For this review, take the finished solid that the model builds, in its own axes (mm). Face numbers are marked on the shaded views. A direction names the side the tool comes from. Round coordinates to 2 decimals unless told otherwise and drop trailing zeros. Order: outer loops, then holes, each group sorted by start corner. A loop starts at its lowest first (then second) coordinate and runs counter-clockwise, first axis right, second up. Notation, with made-up numbers: M 76.5,13 L 117.5,13 A24 cw 117.5,25 Z; hole C -11.75,79 d10. An arc over 180 degrees is marked long. Use a Markdown table: item, result.
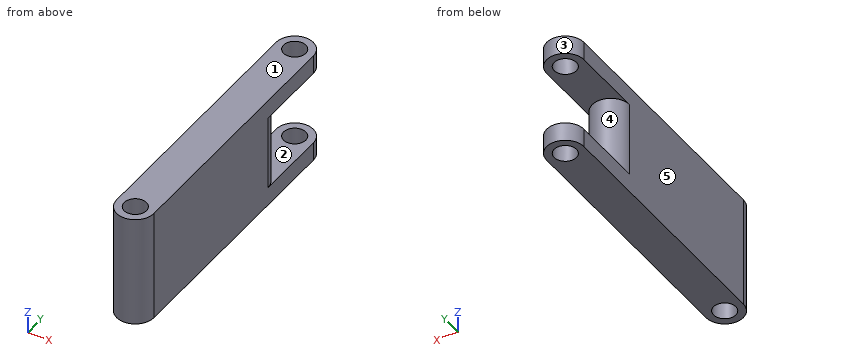
from build123d import *

# Parameters (mm, degrees)
SKETCH1_W           = 12.7
SKETCH1_H           = 101.6
BOSS_EXTRUDE1_DEPTH = 19.05
FILLET2_RADIUS      = 6.35
FILLET2_LENGTH      = 38.1
SKETCH2_R           = 3.81
CUT_EXTRUDE1_DEPTH  = 38.1
FILLET3_RADIUS      = 6.35
FILLET3_LENGTH      = 38.1
SKETCH3_W           = 25.4
SKETCH3_H           = 25.4
CUT_EXTRUDE2_DEPTH  = 56.72102386
FILLET4_RADIUS      = 6.35
FILLET4_LENGTH      = 25.4


with BuildPart() as part:
    # Sketch1 → Boss-Extrude1 (new, symmetric)
    with BuildSketch(Plane.XY):
        Rectangle(SKETCH1_W, SKETCH1_H)
    extrude(amount=BOSS_EXTRUDE1_DEPTH, both=True)

    # Fillet2: full round fillet: the end face becomes a half cylinder, R = half its width
    fillet2_face = Plane((0, -50.8, 0), x_dir=(0, 0, 1), z_dir=(0, -1, 0))  # on the end face: x along it, z out of the body
    fillet2_slab = fillet2_face.offset(-FILLET2_RADIUS / 2) * Box(FILLET2_LENGTH, 2 * FILLET2_RADIUS, FILLET2_RADIUS, mode=Mode.PRIVATE)  # the body's end, R deep
    fillet2_round = Plane((0, -44.45, 0), x_dir=(0, -1, 0), z_dir=(0, 0, 1)) * Cylinder(FILLET2_RADIUS, FILLET2_LENGTH, mode=Mode.PRIVATE)  # its axis R under the face
    add(fillet2_slab - fillet2_round, mode=Mode.SUBTRACT)

    # Sketch2 → Cut-Extrude1 (cut)
    with BuildSketch(Plane.XY.offset(19.05)):
        with Locations((0, -44.45)):
            Circle(SKETCH2_R)
    cut_extrude1 = extrude(amount=-CUT_EXTRUDE1_DEPTH, mode=Mode.SUBTRACT)

    # Mirror3: Cut-Extrude1 across plane
    add(cut_extrude1.mirror(Plane.ZX), mode=Mode.SUBTRACT)

    # Fillet3: full round fillet: the end face becomes a half cylinder, R = half its width
    fillet3_face = Plane((0, 50.8, 0), x_dir=(0, 0, 1), z_dir=(0, 1, 0))  # on the end face: x along it, z out of the body
    fillet3_slab = fillet3_face.offset(-FILLET3_RADIUS / 2) * Box(FILLET3_LENGTH, 2 * FILLET3_RADIUS, FILLET3_RADIUS, mode=Mode.PRIVATE)  # the body's end, R deep
    fillet3_round = Plane((0, 44.45, 0), x_dir=(0, 1, 0), z_dir=(0, 0, 1)) * Cylinder(FILLET3_RADIUS, FILLET3_LENGTH, mode=Mode.PRIVATE)  # its axis R under the face
    add(fillet3_slab - fillet3_round, mode=Mode.SUBTRACT)

    # Sketch3 → Cut-Extrude2 (cut, through all)
    with BuildSketch(Plane.ZY.offset(6.35)):
        with Locations((0, 38.1)):
            Rectangle(SKETCH3_W, SKETCH3_H)
    extrude(amount=-CUT_EXTRUDE2_DEPTH, mode=Mode.SUBTRACT)

    # Fillet4: full round fillet: the end face becomes a half cylinder, R = half its width
    fillet4_face = Plane((0, 25.4, 0), x_dir=(0, 0, -1), z_dir=(0, 1, 0))  # on the end face: x along it, z out of the body
    fillet4_slab = fillet4_face.offset(-FILLET4_RADIUS / 2) * Box(FILLET4_LENGTH, 2 * FILLET4_RADIUS, FILLET4_RADIUS, mode=Mode.PRIVATE)  # the body's end, R deep
    fillet4_round = Plane((0, 19.05, 0), x_dir=(0, 1, 0), z_dir=(0, 0, -1)) * Cylinder(FILLET4_RADIUS, FILLET4_LENGTH, mode=Mode.PRIVATE)  # its axis R under the face
    add(fillet4_slab - fillet4_round, mode=Mode.SUBTRACT)


solid = part.part
Q1. Add section D-D (z = 14.5). Write out the cut boundary in (x, y).
Determined:
| item | result |
|---|---|
| outline | M -6.35,-44.45 A6.35 ccw 6.35,-44.45 L 6.35,44.45 A6.35 ccw -6.35,44.45 Z; hole C 0,-44.45 d7.62; hole C 0,44.45 d7.62 |
Q2. Add section C-C (z = 4). Write out the cut boundary in (x, y), then the cut area to 3 significant figures.
Determined:
| item | result |
|---|---|
| outline | M -6.35,-44.45 A6.35 ccw 6.35,-44.45 L 6.35,19.05 A6.35 ccw -6.35,19.05 Z; hole C 0,-44.45 d7.62 |
| area | 888 mm^2 |
Q3. Wall thickness on line 1 along Y through (x, z) = (0, -16); line 2 along Z through (x, y) = (1, 35); line 3 along Y through (x, z) = (-2.5, -13): over which ranges is each line inside the solid? List them lowest first. Write a range as [from, to].
Determined:
| item | result |
|---|---|
| line 1 | y = [-50.8, -48.26], [-40.64, 40.64], [48.26, 50.8] |
| line 2 | z = [-19.05, -12.7], [12.7, 19.05] |
| line 3 | y = [-50.29, -47.33], [-41.57, 41.57], [47.33, 50.29] |
Q4. Machinability: for the marked faces 4 and 5, which of the approach directions +Z, -Z, +X, -X, +Y, -Y give a long, thin tool a straight path to every point of the face, cutting with its end or side? Answer none if there is none.
Determined:
| item | result |
|---|---|
| face 4 | +Y |
| face 5 | +Z, -Z, -X, +Y, -Y |
Q5. Add section B-B (y = 36.5). Write out the cut boundary in (x, z).
Determined:
| item | result |
|---|---|
| outline | M -6.35,-19.05 L 6.35,-19.05 L 6.35,-12.7 L -6.35,-12.7 Z; M -6.35,12.7 L 6.35,12.7 L 6.35,19.05 L -6.35,19.05 Z |
Q6. Add section A-A (x = 0). Write out the cut boundary in (y, z).
Determined:
| item | result |
|---|---|
| outline | M -50.8,-19.05 L -48.26,-19.05 L -48.26,19.05 L -50.8,19.05 Z; M -40.64,-19.05 L 40.64,-19.05 L 40.64,-12.7 L 25.4,-12.7 L 25.4,12.7 L 40.64,12.7 L 40.64,19.05 L -40.64,19.05 Z; M 48.26,-19.05 L 50.8,-19.05 L 50.8,-12.7 L 48.26,-12.7 Z; M 48.26,12.7 L 50.8,12.7 L 50.8,19.05 L 48.26,19.05 Z |
Q7. Draft analysis for pull direction Z (two halves, no side actions). For the marked faces 1, 2 and 3, state which applies: pulls with the +Z half, pulls with the -Z half, needs draft (parallel to the pull), parting line crosses it, or undercut.
Determined:
| item | result |
|---|---|
| face 1 | pulls with the +Z half |
| face 2 | undercut |
| face 3 | needs draft |
Q8. Clearance check with flat-ended pins moving along their axes: pin 1 (5 mm diameter, centred on x = -3.5, z = -9, fed in from +Y); pin 2 (1.5 mm diameter, centred on x = 1, z = 7, fed in from +Y). State where each tip first meets the part, or that it passes through.
Determined:
| item | result |
|---|---|
| pin 1 | stops at y = 25.32 |
| pin 2 | stops at y = 25.4 |
